CAD build for the part. Positions are in the model's coordinates, mm. A direction names the side the tool comes from. Coordinates: 2 decimals unless noted, no trailing zeros. Loops run counter-clockwise (first coordinate to the right, second up) from the corner with the lowest first, then second, coordinate; pieces in that order, holes last. Notation, with made-up numbers: (-35.5, -20.5) -> (22.5, -20.5) arc R27 cw to (22.5, 5.5) -> close; hole circle Ø7 at (63, 31). An arc over 180 degrees is marked (long way). Answer as a JSON object with one key per item and string values. Group by question number.
from build123d import *

# Parameters (mm, degrees)
SKETCH1_W           = 23.8
SKETCH1_H           = 11.5
BODY_DEPTH          = 20.32
SKETCH2_W           = 4.1
SKETCH2_H           = 11.5
SKETCH2_R           = 1.125
BOSS_EXTRUDE2_DEPTH = 1.5748
SKETCH3_R           = 1.915
BOSS_EXTRUDE3_DEPTH = 6.9215
SKETCH4_R           = 5.75
BOSS_EXTRUDE4_DEPTH = 3.5941


with BuildPart() as part:
    # Sketch1 → Body (new body)
    with BuildSketch(Plane.XY):
        Rectangle(SKETCH1_W, SKETCH1_H)
    extrude(amount=BODY_DEPTH)

    # Sketch2 → Boss-Extrude2 (add)
    with BuildSketch(Plane(origin=(0, 0, 14.732), x_dir=(-1, 0, 0), z_dir=(0, 0, -1))):
        with Locations((13.95, 0)):
            Rectangle(SKETCH2_W, SKETCH2_H)
        with Locations((13.95, 0)):
            Circle(SKETCH2_R, mode=Mode.SUBTRACT)
        with Locations((-13.95, 0)):
            Rectangle(SKETCH2_W, SKETCH2_H)
        with Locations((-13.95, 0)):
            Circle(SKETCH2_R, mode=Mode.SUBTRACT)
    extrude(amount=-BOSS_EXTRUDE2_DEPTH)

    # Sketch3 → Boss-Extrude3 (add)
    with BuildSketch(Plane.XY.offset(20.32)):
        with Locations((6.15, 0)):
            Circle(SKETCH3_R)
    extrude(amount=BOSS_EXTRUDE3_DEPTH)

    # Sketch4 → Boss-Extrude4 (add)
    with BuildSketch(Plane.XY.offset(20.32)):
        with Locations((6.15, 0)):
            Circle(SKETCH4_R)
    extrude(amount=BOSS_EXTRUDE4_DEPTH)


solid = part.part
Item 1: Band-saw the part on B-B, the plane z = 22. List the corners of the cut face in (x, y), and give its area (3 significant figures).
Item 2: Band-saw the part on C-C, the plane y = -1.5. List the corners of the cut face in (x, z).
Item 3: Flat gauge pins, fed straight in: P1, Ø2, axis at y = 2, z = 17.5, coming from the -X side; P2, Ø3, axis at x = 8, z = 24, coming from the +Y side; P3, Ø4.5, axis at x = -13.5, y = 2.5, coming from the +Z side; P4, Ø1.2, axis at x = 14, y = 0, coming from the +Z side. Where does each tip first touch, or does it go through?
Item 4: Band-saw the part on D-D, the plane x = 3. List the corners of the cut face in (y, z).
Item 5: Band-saw the part on A-A, the plane x = 13.95. List the corners of the cut face in (y, z) (3 decimals).
Item 6: Pull direction X, two halves, no side cores. Call faces 5 (the flat face through (0, -5.75, 10)), 6 (the cylindrical face through (12.877, 0.338, 15.508)), 7 (the flat face through (-16, 0, 16)): +X half, -X half, draft (parallel to the pull), parting line (faces both ways), or undercut.
Item 7: Drill centre lines: L1, parallel to Y at x = 13.95, z = 15.95 (3 decimals); L2, parallel to X at y = -2.5, z = 13.5; L3, parallel to Z at x = 2, y = 0.25. Where is each one in solid material? Low to high.
Item 8: 3-axis set-ups, long thin cutter, end or side, ignore diameter. For faces 1 (the flat face through (-11.9, 0, 18)), 2 (the flat face through (14, 1.4, 16.307)), 3 (the flat face through (-13.9, 1.4, 14.732)), 4 (the cylindrical face through (4.237, 0.084, 25.555)): which of +Z, -Z, +X, -X, +Y, -Y reach the whole face in a straight line?
Reply:
{
 "1": {"outline": "circle Ø11.5 at (6.15, 0)", "area": "104 mm²"},
 "2": {"outline": "(-16, 14.73) -> (-11.9, 14.73) -> (-11.9, 0) -> (11.9, 0) -> (11.9, 14.73) -> (16, 14.73) -> (16, 16.31) -> (11.9, 16.31) -> (11.9, 20.32) -> (11.7, 20.32) -> (11.7, 23.91) -> (7.34, 23.91) -> (7.34, 27.24) -> (4.96, 27.24) -> (4.96, 23.91) -> (0.6, 23.91) -> (0.6, 20.32) -> (-11.9, 20.32) -> (-11.9, 16.31) -> (-16, 16.31) -> close"},
 "3": {"P1": "x = -11.9", "P2": "y = 5.74", "P3": "z = 20.32", "P4": "through"},
 "4": {"outline": "(-5.75, 0) -> (5.75, 0) -> (5.75, 20.32) -> (4.81, 20.32) -> (4.81, 23.91) -> (-4.81, 23.91) -> (-4.81, 20.32) -> (-5.75, 20.32) -> close"},
 "5": {"outline": "(-5.75, 14.732) -> (-1.125, 14.732) -> (-1.125, 16.307) -> (-5.75, 16.307) -> close; (1.125, 14.732) -> (5.75, 14.732) -> (5.75, 16.307) -> (1.125, 16.307) -> close"},
 "6": {"face 5": "draft", "face 6": "undercut", "face 7": "-X half"},
 "7": {"L1": "-5.75 to -1.125, 1.125 to 5.75", "L2": "-11.9 to 11.9", "L3": "0 to 23.91"},
 "8": {"face 1": "+Z, -X, +Y, -Y", "face 2": "+Z, +X, +Y, -Y", "face 3": "-Z, -X, +Y, -Y", "face 4": "+Z"}
}
